Here's the drawing with two shaded views (mm, measured from the low corner). I have some questions. Round coordinates to 2 decimals unless told otherwise and drop trailing zeros. Loops run counter-clockwise (first coordinate to the right, second up) from the corner with the lowest first, then second, coordinate; pieces in that order, holes last. Notation, with made-up numbers: M -11,59.5 L 42,59.5 A12 cw 42,69.5 Z; hole C -22,-24 d2. An arc over 180 degrees is marked long. One line per item, written item: value. Start each with the question number.
Q1. Imagine slicing it at C-C (z = 95). Please give me the cut outline in (x, y) (3 decimals), then the cut area to 4 significant figures.
Q2. Imagine slicing it at B-B (z = 4). Please give me the cut outline in (x, y), then the cut area to 3 significant figures.
Q3. Imagine slicing it at A-A (x = 4). Please give me the cut outline in (y, z).
Q4. Imagine slicing it at D-D (y = 0.9). Give the number of separate pieces and of enclosed holes in the cut face, then the cut area to 3 significant figures.
Q5. Please list where these lines run through material, in increasing order: line 1 along Z through (x, y) = (86, 1.25); line 2 along X through (y, z) = (0.95, 196); line 3 along Z through (x, y) = (46.5, 1).
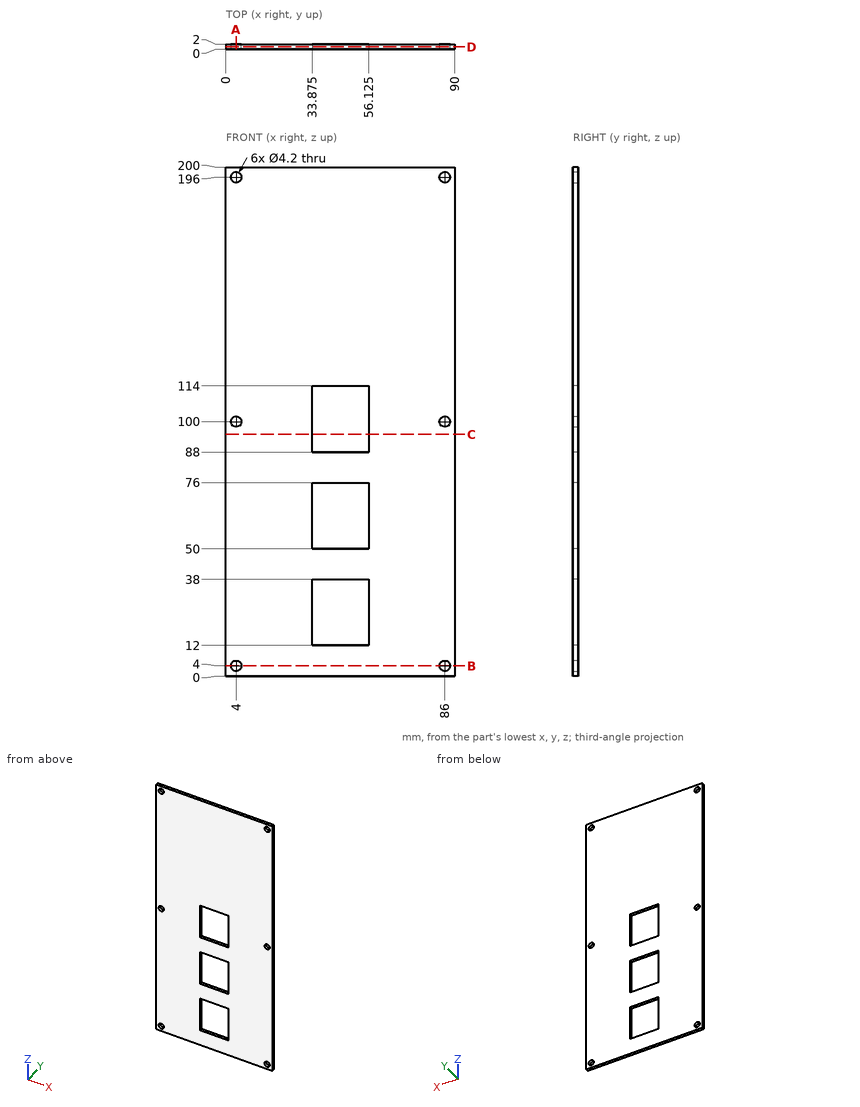
Report:
1. outline: M 0,0 L 33.875,0 L 33.875,2 L 0,2 Z; M 56.125,0 L 90,0 L 90,2 L 56.125,2 Z
1. area: 135.5 mm²
2. outline: M 0,0 L 1.9,0 L 1.9,2 L 0,2 Z; M 6.1,0 L 83.9,0 L 83.9,2 L 6.1,2 Z; M 88.1,0 L 90,0 L 90,2 L 88.1,2 Z
2. area: 163 mm²
3. outline: M 0,0 L 2,0 L 2,1.9 L 0,1.9 Z; M 0,6.1 L 2,6.1 L 2,97.9 L 0,97.9 Z; M 0,102.1 L 2,102.1 L 2,193.9 L 0,193.9 Z; M 0,198.1 L 2,198.1 L 2,200 L 0,200 Z
4. separate pieces: 1
4. enclosed holes: 9
4. area: 16,200 mm²
5. line 1: z = 0 to 1.9, 6.1 to 97.9, 102.1 to 193.9, 198.1 to 200
5. line 2: x = 0 to 1.9, 6.1 to 83.9, 88.1 to 90
5. line 3: z = 0 to 12, 38 to 50, 76 to 88, 114 to 200
